Verification items for the finished model (mm, model axes). A direction names the side the tool comes from. Coordinates: 2 decimals unless noted, no trailing zeros. Loops run counter-clockwise (first coordinate to the right, second up) from the corner with the lowest first, then second, coordinate; pieces in that order, holes last. Notation, with made-up numbers: (44, -13) - (71, -13) arc R23 ccw to (71, 20) - close; hole circle Ø1 at (71.5, 46.25). An arc over 180 degrees is marked (long way). Answer as CSV lines item,"result". Start each with the question number.
1. Gauge pin test, flat ends, axial feed: P1, Ø10, axis at x = -2.5, y = 8, coming from the +Z side; P2, Ø8, axis at x = 15.5, z = -10, coming from the +Y side; P3, Ø2, axis at y = 5, z = 17.5, coming from the +X side. Record the tip position at first contact, or that the pin passes through.
2. Cross-section at A-A (x = 0). Enter the section's corners in (y, z).
3. Material ranges on line 1 (Z direction, x = 0, y = -11.5); line 2 (Z direction, x = 0, y = -4); line 3 (Y direction, x = 17.5, z = 14), recorded low to high. Write a range as [from, to].
4. Cross-section at B-B (y = 7). Enter the section's corners in (x, z), plus the area to 3 significant figures.
5. Cross-section at D-D (y = -12). Enter the section's corners in (x, z), plus the area to 3 significant figures.
6. Set-up check for faces 5 (the flat face through (9.2, -17, 18.3)), 6 (the cylindrical face through (-17, 6, 0)), 7 (the flat face through (17.094, 12.014, 16.959)), 8 (the flat face through (-4, -8, -24)): record each of +Z, -Z, +X, -X, +Y, -Y from which the full face is reachable in a straight line by a thin tool's end or side.
7. Cross-section at C-C (y = -5). Enter the section's corners in (x, z).
8. Release check for a two-part mould opening along Z. For faces 1 (the flat face through (-12, 13, 21)), 2 (the flat face through (6.14, 12.014, -23.284)), 3 (the flat face through (17.971, 5.423, 16.387)), 4 (the flat face through (17.245, 12.014, -17.097)) record: pulls with the +Z half, pulls with the -Z half, needs draft (parallel to the pull), parting line crosses it, or undercut.
Autodesk Inventor part; units mm, degrees
ref_plane "YZ Plane" through (0, 0, 0) normal (1, 0, 0) x (0, 1, 0)
ref_plane "XZ Plane" through (0, 0, 0) normal (0, 1, 0) x (-1, 0, 0)
ref_plane "XY Plane" through (0, 0, 0) normal (0, 0, 1) x (1, 0, 0)
sketch "Sketch1" plane through (0, 0, 0) normal (0, 0, 1) x (1, 0, 0)
  line L0 (-31.4382, 0) -> (-31.4382, -8)
  line L1 (-26.5, -13) -> (-26.5, -17)
  line L2 (-26.5, -17) -> (-20.25, -17)
  line L3 (-20.25, -17) -> (-20.25, -19)
  line L4 (-20.25, -19) -> (-15.25, -19)
  line L5 (-15.25, -19) -> (-15.25, -6.5)
  line L6 (-15.25, -6.5) -> (-16.5, -6.5)
  line L7 (-16.5, -6.5) -> (-16.5, 0)
  line L8 (-26.5, -13) -> (-23.9382, -13)
  line L9 (-31.4382, 0) -> (-16.5, 0)
  line L10 (-37.7259, 0) -> (6.2876, 0)
  line L11 (-31.4382, -8) -> (-23.9382, -8)
  line L12 (-23.9382, -8) -> (-23.9382, -13)
  line L13 (0, -22.8) -> (0, 3.8)
  point P0 (0, 0)
  dimension "d1" = 15.25
  dimension "d2" = 5
  dimension "d3" = 6.25
  dimension "d4" = 2
  dimension "d6" = 4
  dimension "d8" = 8
  dimension "d10" = 6.5
  dimension "d11" = 16.5
  dimension "d12" = 14.9382
  dimension "d14" = 5
  dimension "d15" = 7.5
revolve "Revolution1" add sketch "Sketch1" angle 360 about axis through (0, -10, 0) along (0, 1, 0)
sketch "Sketch2" plane through (0, 0, 0) normal (0, 1, 0) x (1, 0, 0)
  circle A0 centre (0, 0) radius 17 construction
  line L0 (0, 0) -> (-36.8022, 11.7026)
  line L1 (-36.8022, -11.7026) -> (0, 0)
  line L2 (-50.4503, 0) -> (45.0863, 0)
  arc A1 (-16.2006, 5.1516) -> (-16.2006, -5.1516) centre (0, 0) ccw
  circle A2 centre (0, 0) radius 31.4382
  arc A3 (-29.96, 9.5269) -> (-29.96, -9.5269) centre (0, 0) ccw
  line L3 (-29.96, -9.5269) -> (-16.2006, -5.1516)
  line L4 (-29.96, 9.5269) -> (-16.2006, 5.1516)
  dimension "d17" = 34
  dimension "d18" = 35.28
extrude "Extrusion1" add sketch "Sketch2" along normal blind 13 contours A1 L2 A2 L0 | L1 A2 L2 A1
chamfer "Chamfer1" distance 2 angle 45 2 edges at (-23.0803, 13, -7.3392) (-23.0803, 13, 7.3392)
pattern_circular "Circular Pattern1" count 6 over 360 about axis through (0, -10, 0) along (0, 1, 0) of "Extrusion1", "Chamfer1"
fillet "Fillet1" radius 2 2 edges at (31.4382, -8, 0) (26.5, -17, 0)
properties part number "shaft_fixture"
Values follow:
1,P1,"stops at z = 30.71"
1,P2,"stops at y = 11.95"
1,P3,"stops at x = 20.29"
2,outline,"(-19, -20.25) - (-17, -20.25) - (-17, -24.5) arc R2 ccw to (-15, -26.5) - (-13, -26.5) - (-13, -23.94) - (-8, -23.94) - (-8, -29.44) arc R2 ccw to (-6, -31.44) - (0, -31.44) - (0, -16.5) - (-6.5, -16.5) - (-6.5, -15.25) - (-19, -15.25) - close; (-19, 15.25) - (-6.5, 15.25) - (-6.5, 16.5) - (0, 16.5) - (0, 31.44) - (-6, 31.44) arc R2 ccw to (-8, 29.44) - (-8, 23.94) - (-13, 23.94) - (-13, 26.5) - (-15, 26.5) arc R2 ccw to (-17, 24.5) - (-17, 20.25) - (-19, 20.25) - close"
3,line 1,"z = [-23.94, -15.25], [15.25, 23.94]"
3,line 2,"z = [-31.44, -16.5], [16.5, 31.44]"
3,line 3,"y = [-17, 0]"
4,outline,"(-29.96, -9.53) - (-16.2, -5.15) arc R17 cw to (-16.2, 5.15) - (-29.96, 9.53) arc R31.44 ccw to start; (-23.23, -21.18) arc R31.44 ccw to (-6.73, -30.71) - (-3.64, -16.61) arc R17 cw to (-12.56, -11.45) - close; (-23.23, 21.18) - (-12.56, 11.45) arc R17 cw to (-3.64, 16.61) - (-6.73, 30.71) arc R31.44 ccw to start; (3.64, -16.61) - (6.73, -30.71) arc R31.44 ccw to (23.23, -21.18) - (12.56, -11.45) arc R17 cw to start; (3.64, 16.61) arc R17 cw to (12.56, 11.45) - (23.23, 21.18) arc R31.44 ccw to (6.73, 30.71) - close; (16.2, -5.15) - (29.96, -9.53) arc R31.44 ccw to (29.96, 9.53) - (16.2, 5.15) arc R17 cw to start"
4,area,"1,290 mm²"
5,outline,"circle Ø47.88 at (0, 0); hole circle Ø30.5 at (0, 0)"
5,area,"1,070 mm²"
6,face 5,"-Y"
6,face 6,"+Y"
6,face 7,"+X, +Y"
6,face 8,"none"
7,outline,"circle Ø62.88 at (0, 0); hole circle Ø33 at (0, 0)"
8,face 1,"needs draft"
8,face 2,"pulls with the -Z half"
8,face 3,"undercut"
8,face 4,"undercut"
